```python
from build123d import *

# Parameters (mm, degrees)
SKETCH1_W           = 40
SKETCH1_H           = 22
SKETCH1_R           = 4
SKETCH1_R_2         = 1.5
SKETCH1_R_3         = 1
BOSS_EXTRUDE1_DEPTH = 1.5
SKETCH2_W           = 1.5
SKETCH2_H           = 22
BOSS_EXTRUDE2_DEPTH = 36
FILLET1_R           = 1
SKETCH3_R           = 1.5
SKETCH3_R_2         = 1
SKETCH3_W           = 2.75
SKETCH3_H           = 4.25
CUT_EXTRUDE1_DEPTH  = 55.927224579
FILLET2_R           = 1


with BuildPart() as part:
    # Sketch1 → Boss-Extrude1 (new body)
    with BuildSketch(Plane(origin=(0, 0, 0), x_dir=(1, 0, 0), z_dir=(0, 1, 0))):
        Rectangle(SKETCH1_W, SKETCH1_H)
        with Locations(Location((0, 0, 0), (0, 0, 270))):
            Circle(SKETCH1_R, mode=Mode.SUBTRACT)
        with Locations(Location((0, 7, 0), (0, 0, 270))):
            Circle(SKETCH1_R_2, mode=Mode.SUBTRACT)
        with Locations(Location((7, 0, 0), (0, 0, 270))):
            Circle(SKETCH1_R_2, mode=Mode.SUBTRACT)
        with Locations(Location((0, -7, 0), (0, 0, 270))):
            Circle(SKETCH1_R_2, mode=Mode.SUBTRACT)
        with Locations(Location((-7, 0, 0), (0, 0, 270))):
            Circle(SKETCH1_R_2, mode=Mode.SUBTRACT)
        with Locations(Location((5, 5, 0), (0, 0, 270))):
            Circle(SKETCH1_R_3, mode=Mode.SUBTRACT)
        with Locations(Location((5, -5, 0), (0, 0, 270))):
            Circle(SKETCH1_R_3, mode=Mode.SUBTRACT)
        with Locations(Location((-5, -5, 0), (0, 0, 270))):
            Circle(SKETCH1_R_3, mode=Mode.SUBTRACT)
        with Locations(Location((-5, 5, 0), (0, 0, 270))):
            Circle(SKETCH1_R_3, mode=Mode.SUBTRACT)
    extrude(amount=BOSS_EXTRUDE1_DEPTH)

    # Sketch2 → Boss-Extrude2 (add)
    with BuildSketch(Plane(origin=(0, 0, 0), x_dir=(-1, 0, 0), z_dir=(0, -1, 0))):
        with Locations((-19.25, 0)):
            Rectangle(SKETCH2_W, SKETCH2_H)
    boss_extrude2 = extrude(amount=BOSS_EXTRUDE2_DEPTH)

    # Mirror1: Boss-Extrude2 across plane
    add(boss_extrude2.mirror(Plane(origin=(0, 0, 0), x_dir=(0, 0, 1), z_dir=(1, 0, 0))))

    # Fillet1
    fillet1_edges = [part.edges().sort_by_distance(p)[0] for p in [
        (-20, 1.5, 0),
        (20, 1.5, 0),
    ]]
    fillet(fillet1_edges, radius=FILLET1_R)

    # Sketch3 → Cut-Extrude1 (cut, through all)
    with BuildSketch(Plane.ZY.offset(20)):
        with Locations((0, -7.5)):
            Circle(SKETCH3_R)
        with Locations((0, -24.75)):
            Circle(SKETCH3_R_2)
        with Locations((-7, -31.75)):
            Circle(SKETCH3_R_2)
        with Locations((7, -31.75)):
            Circle(SKETCH3_R_2)
        with BuildLine():
            Line((-4, -31.75), (-4, -36))
            Line((-4, -36), (4, -36))
            Line((4, -36), (4, -31.75))
            ThreePointArc((4, -31.75), (0, -27.75), (-4, -31.75))
        make_face()
        with Locations((-4.125, -14.625)):
            Rectangle(SKETCH3_W, SKETCH3_H)
        with Locations((3.625, -14.625)):
            Rectangle(SKETCH3_W, SKETCH3_H)
    extrude(amount=-CUT_EXTRUDE1_DEPTH, mode=Mode.SUBTRACT)

    # Fillet2
    fillet2_edges = [part.edges().sort_by_distance(p)[0] for p in [
        (-19.25, -36, -4),
        (-19.25, -36, 4),
        (19.25, -36, 4),
        (19.25, -36, -4),
        (19.25, -36, 11),
        (19.25, -36, -11),
        (-19.25, -36, -11),
        (-19.25, -36, 11),
    ]]
    fillet(fillet2_edges, radius=FILLET2_R)


solid = part.part
```
Check sheet for the modelled part. Datum: model origin and axes. Units: mm. A direction names the side the tool comes from. Coordinates: 2 decimals unless noted, no trailing zeros. Write each loop counter-clockwise with the first axis right and the second up, starting at its lowest first coordinate (ties: lowest second). Pieces come first, ordered by that corner, then holes. Notation, with made-up numbers: (83, -28) -> (90, -28) arc R12 cw to (90, -5) -> close; hole circle Ø2 at (43.25, -27.75). An arc over 180 degrees is marked (long way). Use a Markdown table: item, result.
1. Sectioned sample at B-B (y = -19). Enter the section's corners in (x, z), plus the area to 3 significant figures.
Reported:
| item | result |
|---|---|
| outline | (-20, -11) -> (-18.5, -11) -> (-18.5, 11) -> (-20, 11) -> close; (18.5, -11) -> (20, -11) -> (20, 11) -> (18.5, 11) -> close |
| area | 66.0 mm2 |
2. Sectioned sample at C-C (z = 7). Enter the section's corners in (x, y), plus the area to 3 significant figures.
Reported:
| item | result |
|---|---|
| outline | (-20, -36) -> (-18.5, -36) -> (-18.5, -32.75) -> (-20, -32.75) -> close; (-20, -30.75) -> (-18.5, -30.75) -> (-18.5, 0) -> (-1.5, 0) -> (-1.5, 1.5) -> (-19, 1.5) arc R1 ccw to (-20, 0.5) -> close; (1.5, 0) -> (18.5, 0) -> (18.5, -30.75) -> (20, -30.75) -> (20, 0.5) arc R1 ccw to (19, 1.5) -> (1.5, 1.5) -> close; (18.5, -36) -> (20, -36) -> (20, -32.75) -> (18.5, -32.75) -> close |
| area | 157 mm2 |
3. Go/stop test with a flat-tipped pin: pin 1 Ø0.8 at (x, z) = (19, -4) entering from -Y. Record where the tip stops, or that it passes through.
Reported:
| item | result |
|---|---|
| pin 1 | stops at y = -35.8 |
4. Sectioned sample at A-A (x = -5). Enter the section's corners in (y, z), plus the area to 3 significant figures.
Reported:
| item | result |
|---|---|
| outline | (0, -11) -> (1.5, -11) -> (1.5, -6) -> (0, -6) -> close; (0, -4) -> (1.5, -4) -> (1.5, 4) -> (0, 4) -> close; (0, 6) -> (1.5, 6) -> (1.5, 11) -> (0, 11) -> close |
| area | 27.0 mm2 |
5. Scan lines: line 1 along X through (y, z) = (-1.5, 0); line 2 along X through (y, z) = (0.9, 5); line 3 along Y through (x, z) = (1, -4). Record each from-to range of solid material in increasing order.
Reported:
| item | result |
|---|---|
| line 1 | x = -20 to -18.5, 18.5 to 20 |
| line 2 | x = -19.92 to -6, -4 to 4, 6 to 19.92 |
| line 3 | y = 0 to 1.5 |
6. Sectioned sample at D-D (y = -13.5). Enter the section's corners in (x, z).
Reported:
| item | result |
|---|---|
| outline | (-20, -11) -> (-18.5, -11) -> (-18.5, -5.5) -> (-20, -5.5) -> close; (-20, -2.75) -> (-18.5, -2.75) -> (-18.5, 2.25) -> (-20, 2.25) -> close; (-20, 5) -> (-18.5, 5) -> (-18.5, 11) -> (-20, 11) -> close; (18.5, -11) -> (20, -11) -> (20, -5.5) -> (18.5, -5.5) -> close; (18.5, -2.75) -> (20, -2.75) -> (20, 2.25) -> (18.5, 2.25) -> close; (18.5, 5) -> (20, 5) -> (20, 11) -> (18.5, 11) -> close |
7. Tool access check on faces 1 (the cylindrical face through (19.699, 1.215, -0.154)), 2 (the flat face through (-19, -16.75, 4)), 3 (the flat face through (18.5, -18, 0)), 4 (the cylindrical face through (-19.24, -35.715, -4.301)). Record the directions out of +Z, -Z, +X, -X, +Y, -Y that give a thin tool (end or side, any length) a straight path to the whole face; none if there is none.
Reported:
| item | result |
|---|---|
| face 1 | +Z, -Z, +X, +Y |
| face 2 | +X, -X |
| face 3 | +Z, -Z, -Y |
| face 4 | +X, -X, -Y |
8. Release check for a two-part mould opening along Y. For faces 5 (the flat face through (-19, -16.75, -4)), 6 (the flat face through (19, -33, -4)), 7 (the cylindrical face through (-19.24, -35.699, 4.285)), 8 (the cylindrical face through (19.24, -30.76, 6.87)) record: pulls with the +Y half, pulls with the -Y half, needs draft (parallel to the pull), parting line crosses it, or undercut.
Reported:
| item | result |
|---|---|
| face 5 | undercut |
| face 6 | needs draft |
| face 7 | pulls with the -Y half |
| face 8 | undercut |
